from build123d import *

# Parameters (mm, degrees)
F1_DEPTH = 25.4
F3_DEPTH = 25.4
F5_DEPTH = 25.4


with BuildPart() as f1:
    # F0 (on Top) → F1 (new body)
    with BuildSketch(Plane.XY):
        with BuildLine():
            add(Edge.make_bspline(
                [(4.8407731435, 67.5330671062), (3.2844063816, 72.5791703322), (1.6407490349, 75.497781723), (0, 75.4938647151)],
                knots=[0.9332536986, 0.9332536986, 0.9332536986, 0.9332536986, 1, 1, 1, 1], degree=3))
            add(Edge.make_bspline(
                [(0, 75.4938647151), (-1.3704474219, 75.4905930061), (-2.7388658469, 73.4484060128), (-4.0536261968, 69.8308353891)],
                knots=[0, 0, 0, 0, 0.0557503279, 0.0557503279, 0.0557503279, 0.0557503279], degree=3))
            add(Edge.make_bspline(
                [(-4.0536261968, 69.8308353891), (-12.9127091312, 45.455018016), (-19.3355556664, -50.4479074799), (-7.5271204114, -76.0682523251)],
                knots=[0.0557503279, 0.0557503279, 0.0557503279, 0.0557503279, 0.4314056924, 0.4314056924, 0.4314056924, 0.4314056924], degree=3))
            add(Edge.make_bspline(
                [(-7.5271204114, -76.0682523251), (-3.2133106681, -85.4277729417), (3.5335683384, -85.4076795144), (7.8285336494, -76.0217905045)],
                knots=[0.4314056924, 0.4314056924, 0.4314056924, 0.4314056924, 0.5686385887, 0.5686385887, 0.5686385887, 0.5686385887], degree=3))
            add(Edge.make_bspline(
                [(7.8285336494, -76.0217905045), (19.2398591449, -51.0843517129), (13.3427399346, 39.9677122684), (4.8407731435, 67.5330671062)],
                knots=[0.5686385887, 0.5686385887, 0.5686385887, 0.5686385887, 0.9332536986, 0.9332536986, 0.9332536986, 0.9332536986], degree=3))
        make_face()
        with BuildLine():
            add(Edge.make_bspline(
                [(0, 75.4938647151), (-1.3704474219, 75.4905930061), (-2.7388658469, 73.4484060128), (-4.0536261968, 69.8308353891)],
                knots=[0, 0, 0, 0, 0.0557503279, 0.0557503279, 0.0557503279, 0.0557503279], degree=3))
            add(Edge.make_bspline(
                [(4.8407731435, 67.5330671062), (3.2844063816, 72.5791703322), (1.6407490349, 75.497781723), (0, 75.4938647151)],
                knots=[0.9332536986, 0.9332536986, 0.9332536986, 0.9332536986, 1, 1, 1, 1], degree=3))
            Line((4.8407731435, 67.5330671062), (10.3095113427, 128.0233865251))
            Line((10.3095113427, 128.0233865251), (-4.0536261968, 69.8308353891))
        make_face()
        Polygon((-44.0284609795, 128.0233865251), (-4.0536261968, 69.8308353891), (10.3095113427, 128.0233865251), align=None)
        Polygon((10.3095113427, 128.0233865251), (4.8407731435, 67.5330671062), (65.4755681753, 128.0233865251), align=None)
        with BuildLine():
            add(Edge.make_bspline(
                [(-7.5271204114, -76.0682523251), (-3.2133106681, -85.4277729417), (3.5335683384, -85.4076795144), (7.8285336494, -76.0217905045)],
                knots=[0.4314056924, 0.4314056924, 0.4314056924, 0.4314056924, 0.5686385887, 0.5686385887, 0.5686385887, 0.5686385887], degree=3))
            Line((-7.5271204114, -76.0682523251), (-7.5271204114, -118.7840104103))
            Line((-7.5271204114, -118.7840104103), (7.8285336494, -76.0217905045))
        make_face()
        Polygon((-44.0284609795, 128.0233865251), (10.3095113427, 128.0233865251), (65.4755681753, 128.0233865251), (0, 174.2165982723), align=None)
    extrude(amount=F1_DEPTH)

    # F2 (on Front) → F3 (join)
    with BuildSketch(Plane.XZ):
        Polygon((35.0647498421, 65.5660423193), (28.9218947291, 71.0850805044), (22.1357589616, 75.7906955304), (14.8133639544, 79.6086770372), (7.070188251, 82.4788131758), (-0.9716536423, 84.3558401847), (-9.1853370747, 85.2101562267), (-17.441327352, 85.0282882275), (-25.6094225756, 83.8131043541), (-33.5608070045, 81.583768782), (-41.1700825562, 78.375439465), (-48.3172464097, 74.2387136729), (-54.8895835217, 69.2388300428), (-60.7834442096, 63.4546397261), (-65.9058787697, 56.9773628595), (-70.1761033488, 49.9091499686), (-73.5267739546, 42.3614709929), (-75.9050485099, 34.4533573387), (-77.2734202043, 26.3095246824), (-77.6103089988, 18.0584061299), (-76.9104019558, 9.8301267496), (-75.1847370275, 1.7544514229), (-72.4605289807, -6.0412616263), (-68.7807402035, -13.4340693463), (-64.2034031634, -20.307382743), (-58.8007051997, -26.5528055582), (-52.6578500867, -32.0718437433), (-45.8717143191, -36.7774587693), (-38.5493193119, -40.5954402761), (-30.8061436085, -43.4655764147), (-22.7643017153, -45.3426034236), (-14.5506182828, -46.1969194657), (-6.2946280055, -46.0150514664), (1.8734672181, -44.799867593), (9.8248516469, -42.5705320209), (17.4341271986, -39.3622027039), (24.5812910522, -35.2254769118), (31.1536281641, -30.2255932817), (37.047488852, -24.441402965), (42.1699234121, -17.9641260984), (46.4401479913, -10.8959132075), (49.790818597, -3.3482342318), (52.1690931524, 4.5598794223), (53.5374648468, 12.7037120787), (53.8743536413, 20.9548306312), (53.1744465983, 29.1831100115), (51.4487816699, 37.2587853382), (48.7245736231, 45.0544983874), (45.044784846, 52.4473061074), (40.4674478058, 59.320619504), align=None)
        Polygon((-9.1853370747, 85.2101562267), (-0.9716536423, 84.3558401847), (0, 102.0670607686), (-25.6094225756, 83.8131043541), (-17.441327352, 85.0282882275), align=None)
        Polygon((-33.5608070045, 81.583768782), (-25.6094225756, 83.8131043541), (-25.6094225756, 90.1521965861), align=None)
        Polygon((-41.1700825562, 78.375439465), (-33.5608070045, 81.583768782), (-33.5608070045, 90.1521965861), (-48.3172464097, 74.2387136729), align=None)
        Polygon((-54.8895835217, 69.2388300428), (-48.3172464097, 74.2387136729), (-48.3172464097, 83.6073234677), align=None)
    extrude(amount=F3_DEPTH)

    # F4 (on Right) → F5 (join)
    with BuildSketch(Plane.YZ):
        Polygon((-305.4965734482, 58.7429665029), (-183.2486838102, 24.4857445359), (-215.6980782747, 79.0661200881), align=None)
        Polygon((-215.6980782747, 79.0661200881), (-183.2486838102, 24.4857445359), (0, 0), (-50.8633553982, 39.6590679884), align=None)
    extrude(amount=F5_DEPTH)


solid = f1.part
Part model, mm, in its own coordinate system. A direction names the side the tool comes from. Coordinates: 2 decimals unless noted, no trailing zeros. Order: outer loops, then holes, each group sorted by start corner. A loop starts at its lowest first (then second) coordinate and runs counter-clockwise, first axis right, second up. Notation, with made-up numbers: M 84,-40 L 92,-40 A27 ccw 92,-20 Z; hole C 4.25,-38 d6. An arc over 180 degrees is marked long. Use a Markdown table: item, result.
(1) Cut at B-B on y = 104. Write the cut outline in (x, z), then the cut area to 3 significant figures.
A:
| item | result |
|---|---|
| outline | M -27.53,0 L 41.39,0 L 41.39,25.4 L -27.53,25.4 Z |
| area | 1,750 mm^2 |
(2) Flat gauge pins, fed straight in: pin 1 (14 mm diameter, centred on x = 3, y = -56, fed in from -Z); pin 2 (20.5 mm diameter, centred on y = -98, z = 10, fed in from -X); pin 3 (5 mm diameter, centred on x = 26.5, z = 56.5, fed in from +Y). Where does each tip first touch, or does it go through?
A:
| item | result |
|---|---|
| pin 1 | stops at z = 0 |
| pin 2 | stops at x = -7.53 |
| pin 3 | stops at y = 0 |
(3) Pull direction Y, two halves, no side cores. Call faces 1 (the flat face through (-76.06, -12.52, 5.85)), 2 (the flat face through (33.196, 150.797, 12.522)), 3 (the flat face through (12.522, -259.969, 69.047)), 4 (the flat face through (12.522, -40.783, 31.799)): released by +Y, released by -Y, zero draft, split by the parting line, or undercut.
A:
| item | result |
|---|---|
| face 1 | zero draft |
| face 2 | released by +Y |
| face 3 | released by -Y |
| face 4 | undercut |
(4) Probe L1, parallel to Y at x = -8, z = 37.5; L2, parallel to Z at x = -5, y = -77; L3, parallel to X at y = -53.5, z = 1. List the from-to ranges inside material, lowest first.
A:
| item | result |
|---|---|
| L1 | y = -25.4 to 0 |
| L2 | z = 0 to 25.4 |
| L3 | x = -12.54 to 12.79 |
(5) Tool access for faces 5 (the flat face through (50.963, -12.522, 0.55)), 6 (the flat face through (-0.493, -12.522, 93.087)), 7 (the flat face through (-51.56, -12.52, 76.52)), 8 (the flat face through (25.4, -167, 42)): list every direction of +Z, -Z, +X, -X, +Y, -Y with a clear straight run to the whole face (end or side of a thin tool).
A:
| item | result |
|---|---|
| face 5 | -Z, +X, -Y |
| face 6 | +X, +Y, -Y |
| face 7 | +Z, -X, +Y, -Y |
| face 8 | +Z, -Z, +X, -Y |
(6) Cut at A-A on y = -135.5. Write the cut outline in (x, z), then the cut area to 3 significant figures.
A:
| item | result |
|---|---|
| outline | M 0,18.11 L 25.4,18.11 L 25.4,59.89 L 0,59.89 Z |
| area | 1,060 mm^2 |
